Autodesk Fusion 360 part; units mm, degrees
sketch "Sketch1" plane through (0, 0, 0) normal (0, 1, 0) x (1, 0, 0)
  circle A0 centre (0, 0) radius 8.1
  circle A1 centre (0, 0) radius 11.5
  dimension "d1" = 16.2
  dimension "d2" = 23
extrude "Extrude1" add sketch "Sketch1" along normal blind 8 from surface at 2
extrude "Extrude2" add sketch "Sketch1" along normal blind 4 from surface at 10 contours A0 | A1
sketch "Sketch2" plane through (0, 0, 0) normal (0, 0, 1) x (1, 0, 0)
  ellipse E0 centre (0, 24) end of major axis (0, 31.5) minor radius 3.5
  line L0 (0, 16.5) -> (0, 31.5)
  line L1 (3.5, 24) -> (-3.5, 24)
  dimension "d8" = 15
  dimension "d9" = 7
  dimension "d10" = 24
sketch "Sketch3" plane through (0, 0, 0) normal (0, 0, 1) x (1, 0, 0)
  line L0 (6, 12) -> (-6, 12)
  line L1 (-6, 12) -> (-6, 35)
  line L2 (-6, 35) -> (6, 35)
  line L3 (6, 35) -> (6, 12)
  line L4 (6, 12) -> (-6, 35) construction
  line L5 (-6, 12) -> (6, 35) construction
  point P0 (0, 23.5)
  dimension "d11" = 12
  dimension "d12" = 23
  dimension "d13" = 12
extrude "Extrude3" add sketch "Sketch3" along normal mid plane 8
extrude "Extrude4" cut sketch "Sketch2" along normal mid plane 20
fillet "Fillet1" radius 2 8 edges at (6, 24.5, 4) (6, 24.5, -4) (0, 35, 4) (0, 35, -4) (6, 35, 0) (-6, 35, 0) (-6, 24.5, 4) (-6, 24.5, -4)
ref_plane "WorkPlane1" through (0, 10, 0) normal (0, -1, 0) x (-1, 0, 0)
Can you work these out from the model? Positions are in its coordinate system, mm. A direction names the side the tool comes from. Coordinates: 2 decimals unless noted, no trailing zeros. Loops run counter-clockwise (first coordinate to the right, second up) from the corner with the lowest first, then second, coordinate; pieces in that order, holes last. Notation, with made-up numbers: M 82,89 L 119,89 A18 cw 119,96 Z; hole C 11.25,84 d2. An arc over 180 degrees is marked long. Answer as CSV lines item,"result". Start each with the question number.
1. Suppose I cut it at C-C, the plane x = -4.5. List the corners of the cut face in (y, z) for me, plus the area to 3 significant figures.
2. Thinking about a two-plate mould opening in X: for faces 1 (the face through (5.43, 23.37, 3.4)), 2 (the face through (0, 10, 0)), 3 (the face through (0, 35, 0)), which applies, +X half, -X half, draft (parallel to the pull), parting line (faces both ways), or undercut?
3. Suppose I cut it at B-B, the plane y = 7. List the corners of the cut face in (x, z) for me.
4. For faces 4 (the face through (3.5, 21.5, 4)), 5 (the face through (-5.43, 23.63, 3.4)), 6 (the face through (0, 14, 5)), 7 (the face through (6, 24, 0)), 8 (the face through (-1.756, 5.944, -7.907)), which set-ups out of +Z, -Z, +X, -X, +Y, -Y let a thin tool reach every point of the face, with its end or its side?
5. For pin 1 Ø4 at (x, y) = (0.5, 22.5) entering from -Z; pin 2 Ø8 at (x, z) = (3, -2) entering from -Y; pin 3 Ø10 at (x, y) = (-7, 12) entering from -Z; pin 4 Ø8 at (x, y) = (-6, 8) entering from +Z, each with a flat end and sliding along its axis, tell me the tip position at first contact or that it passes through.
6. Suppose I cut it at A-A, the plane z = 7.5. List the corners of the cut face in (x, y) for me.
7. If I drill on probe 1 along X at (y, z) = (5, 0); probe 2 along Y at (x, z) = (-1, 4.75), over which ranges is the centre line in solid material (lowest first)? Write a range as [from, to].
8. Suppose I cut it at D-D, the plane y = 12. List the corners of the cut face in (x, z) for me, plus the area to 3 significant figures.
Output:
1,outline,"M 2,-10.58 L 14,-10.58 L 14,-3.94 L 33,-3.94 A1.94 ccw 34.94,-2 L 34.94,2 A1.94 ccw 33,3.94 L 14,3.94 L 14,10.58 L 2,10.58 L 2,6.73 L 10,6.73 L 10,-6.73 L 2,-6.73 Z"
1,area,"309 mm^2"
2,face 1,"+X half"
2,face 2,"undercut"
2,face 3,"draft"
3,outline,"C 0,0 d23; hole C 0,0 d16.2"
4,face 4,"+Z, +X, -X, +Y"
4,face 5,"+Z, -X, +Y"
4,face 6,"+Y"
4,face 7,"+Z, -Z, +X, +Y"
4,face 8,"-Y"
5,pin 1,"passes through"
5,pin 2,"stops at y = 10"
5,pin 3,"stops at z = -11.32"
5,pin 4,"stops at z = 11.32"
6,outline,"M -8.72,2 L -3.06,2 L -3.06,10 L 3.06,10 L 3.06,2 L 8.72,2 L 8.72,14 L -8.72,14 Z"
7,probe 1,"x = [-11.5, -8.1], [8.1, 11.5]"
7,probe 2,"y = [10, 14]"
8,outline,"C 0,0 d23"
8,area,"415 mm^2"
